from build123d import *

# Parameters (mm, degrees)
F1_DEPTH  = 125
F4_DEPTH  = 2
F10_R     = 9
F11_DEPTH = 25


with BuildPart() as f1:
    # F0 (on Right) → F1 (new body)
    with BuildSketch(Plane.YZ):
        Polygon((179, 0), (0, 0), (0, -2), (177, -2), (177, -30), (179, -30), align=None)
        Polygon((0, -2), (0, 0), (-179, 0), (-179, -30), (-177, -30), (-177, -2), align=None)
    extrude(amount=F1_DEPTH)

    # F3 (on offset) → F4 (join)
    with BuildSketch(Plane.YZ.offset(125)):
        Polygon((179, 0), (0, 0), (-179, 0), (-179, -30), (179, -30), align=None)
    extrude(amount=-F4_DEPTH)

    # F8: sweep along a path in F7
    with BuildLine(Plane.XY.offset(-15)) as f8_path:
        Line((125, 100), (175, 100))
        Line((175, 100), (175, -100))
        Line((175, -100), (125, -100))
    # F5 (on offset) → F8 (sweep)
    with BuildSketch(Plane.YZ.offset(125)):
        with BuildLine():
            ThreePointArc((95, -15), (100, -20), (105, -15))
            ThreePointArc((105, -15), (100, -10), (95, -15))
        make_face()
    sweep(path=f8_path.line, transition=Transition.RIGHT)

    # F9: F1 across face


with BuildPart() as f1_1:
    add(f1.part)
    add(f1.part.mirror(Plane(origin=(0, 0, -3.0289855072), x_dir=(0, 1, 0), z_dir=(-1, 0, 0))))

    # F10 (on Top) → F11 (cut)
    with BuildSketch(Plane.XY):
        Circle(F10_R)
    extrude(amount=-F11_DEPTH, mode=Mode.SUBTRACT)


solid = f1_1.part
Read the model definition and answer for the solid it produces. Units are mm, in the model's axes. A direction names the side the tool comes from. Give positions to 0.01 mm unless a question says otherwise; leave off trailing zeros. Loops run counter-clockwise (first coordinate to the right, second up) from the corner with the lowest first, then second, coordinate; pieces in that order, holes last. Notation, with made-up numbers: (-21.75, -20) -> (4.25, -20) arc R21 cw to (4.25, -10) -> close; hole circle Ø1 at (85, 74). An arc over 180 degrees is marked (long way). Use a Markdown table: item, result.
Q1. Section A-A, the plane y = -54 is taken. Determine the outline of the cut face in (x, z), then the cut area to 3 significant figures.
Solved:
| item | result |
|---|---|
| outline | circle Ø10 at (-175, -15); (-125, -30) -> (-123, -30) -> (-123, -2) -> (123, -2) -> (123, -30) -> (125, -30) -> (125, 0) -> (-125, 0) -> close; circle Ø10 at (175, -15) |
| area | 769 mm^2 |
Q2. Find the intervals of material crossed by line 1 along X through (y, z) = (59.5, -14.5); line 2 along X through (y, z) = (-134.5, -10.75); line 3 along Y through (x, z) = (0, -1), in increasing order.
Solved:
| item | result |
|---|---|
| line 1 | x = -179.97 to -170.03, -125 to -123, 123 to 125, 170.03 to 179.97 |
| line 2 | x = -125 to -123, 123 to 125 |
| line 3 | y = -179 to -9, 9 to 179 |
Q3. A tool of negligible diameter and unlimited length cuts with its end or side. For faces 1 (the face through (2, -177, -16)), 2 (the face through (2, -179, -15)), 3 (the face through (-152.115, -104.619, -16.915)), from which of +Z, -Z, +X, -X, +Y, -Y can it reach the whole face along a straight path? Write none if from no direction.
Solved:
| item | result |
|---|---|
| face 1 | -Z |
| face 2 | +Z, -Z, +X, -X, -Y |
| face 3 | none |
Q4. Each of these flat-tipped pins is pushed along its axis until it touches: pin 1 (8 mm diameter, centred on y = 5.5, z = -7, fed in from +X); pin 2 (6 mm diameter, centred on x = -75, y = 110.5, fed in from -Z); pin 3 (1 mm diameter, centred on y = 4.5, z = -9, fed in from -X). Where does it stop, or does it pass through?
Solved:
| item | result |
|---|---|
| pin 1 | stops at x = 178 |
| pin 2 | stops at z = -2 |
| pin 3 | stops at x = -125 |
Q5. Section D-D, the plane y = 140.5 is taken. Determine the outline of the cut face in (x, z).
Solved:
| item | result |
|---|---|
| outline | (-125, -30) -> (-123, -30) -> (-123, -2) -> (123, -2) -> (123, -30) -> (125, -30) -> (125, 0) -> (-125, 0) -> close |
Q6. Determine the mould class of faces 4 (the face through (30, 3, 0)), 5 (the face through (-171, -1, -18)), 6 (the face through (2, 179, -15)) for opening direction Y: pulls with the +Y half, pulls with the -Y half, needs draft (parallel to the pull), parting line crosses it, or undercut.
Solved:
| item | result |
|---|---|
| face 4 | needs draft |
| face 5 | undercut |
| face 6 | pulls with the +Y half |
Q7. Section C-C, the plane x = 42 is taken. Determine the outline of the cut face in (y, z).
Solved:
| item | result |
|---|---|
| outline | (-179, -30) -> (-177, -30) -> (-177, -2) -> (177, -2) -> (177, -30) -> (179, -30) -> (179, 0) -> (-179, 0) -> close |
Q8. Section B-B, the plane z = -15 is taken. Determine the outline of the cut face in (x, y), then the cut area to 3 significant figures.
Solved:
| item | result |
|---|---|
| outline | (-180, -105) -> (-125, -105) -> (-125, -179) -> (125, -179) -> (125, -105) -> (180, -105) -> (180, 105) -> (125, 105) -> (125, 179) -> (-125, 179) -> (-125, 105) -> (-180, 105) -> close; hole (-170, -95) -> (-125, -95) -> (-125, 95) -> (-170, 95) -> close; hole (-123, -177) -> (123, -177) -> (123, 177) -> (-123, 177) -> close; hole (125, -95) -> (170, -95) -> (170, 95) -> (125, 95) -> close |
| area | 8,420 mm^2 |
